Here's how the part is built. I have some questions about the finished solid (model axes, mm). Give positions to 0.01 mm unless a question says otherwise; leave off trailing zeros. Loops run counter-clockwise (first coordinate to the right, second up) from the corner with the lowest first, then second, coordinate; pieces in that order, holes last. Notation, with made-up numbers: (39, -29.75) - (83, -29.75) arc R5 ccw to (83, -24.75) - close; hole circle Ø5 at (29, -10). An arc over 180 degrees is marked (long way). Return JSON: item names as keys, results as strings. Group by question number.
(1) If we section it at A-A (y = -3.5): Please give me the cut outline in (x, z) (3 decimals), then the cut area to 3 significant figures.
(2) For P1, Ø1.5, axis at x = 4.5, y = -7.5, coming from the -Z side; P2, Ø6, axis at x = -8.5, z = -23.5, coming from the +Y side; P3, Ø1.5, axis at x = -46, y = -8.5, coming from the +Z side, each with a flat end and sliding along its axis, tell me the tip position at first contact or that it passes through.
(3) I need wall thicknesses on probe 1 along Y at (x, z) = (-4, 11); probe 2 along X at (y, z) = (-9.5, 8.5); probe 3 along Z at (x, y) = (-50, -1). Which ranges of each line are inside material? Lowest first, please. Write a range as [from, to].
```python
from build123d import *

# Parameters (mm, degrees)
F0_R     = 73.025
F1_DEPTH = 12.7
F2_R     = 5.08
F4_DEPTH = 0.0254


with BuildPart() as f1:
    # F0 (on Front) → F1 (new body)
    with BuildSketch(Plane.XZ):
        Circle(F0_R)
    extrude(amount=F1_DEPTH)

    # F2
    f2_edges = [f1.edges().sort_by_distance(p)[0] for p in [
        (-73.025, -12.7, 0),
    ]]
    fillet(f2_edges, radius=F2_R)

    # F3 (on face) → F4 (join)
    with BuildSketch(Plane(origin=(0, 0, 0), x_dir=(-1, 0, 0), z_dir=(0, 1, 0))):
        with BuildLine():
            ThreePointArc((-73.025, 0), (-70.485, -2.54), (-67.945, 0))
            ThreePointArc((-67.945, 0), (-70.485, 2.54), (-73.025, 0))
        make_face()
    extrude(amount=F4_DEPTH)


solid = f1.part
```
Values:
{
 "1": {"outline": "circle Ø146.05 at (0, 0)", "area": "16,800 mm2"},
 "2": {"P1": "z = -72.93", "P2": "y = 0", "P3": "z = 57.24"},
 "3": {"probe 1": "[-12.7, 0]", "probe 2": "[-72.17, 72.17]", "probe 3": "[-53.22, 53.22]"}
}
